Autodesk Inventor part; units mm, degrees
ref_plane "YZ Plane" through (0, 0, 0) normal (1, 0, 0) x (0, 1, 0)
ref_plane "XZ Plane" through (0, 0, 0) normal (0, 1, 0) x (-1, 0, 0)
ref_plane "XY Plane" through (0, 0, 0) normal (0, 0, 1) x (1, 0, 0)
sketch "Sketch1" plane through (0, 0, 0) normal (0, 0, 1) x (1, 0, 0)
  line L0 (-12.7, 4.7625) -> (38.1, 4.7625)
  line L1 (-15.875, -9.525) -> (44.45, -9.525)
  line L2 (-19.05, -1.5875) -> (-19.05, -26.8352)
  line L3 (44.45, -1.5875) -> (44.45, -30.4886)
  line L4 (-19.05, -9.525) -> (-15.875, -9.525)
  arc A0 (-12.7, 4.7625) -> (-19.05, -1.5875) centre (-12.7, -1.5875) ccw
  arc A1 (44.45, -1.5875) -> (38.1, 4.7625) centre (38.1, -1.5875) ccw
  line L5 (-19.05, -26.8352) -> (-19.05, -57.15)
  line L6 (-6.0043, -64.9352) -> (31.4043, -64.9352)
  line L7 (44.45, -57.15) -> (44.45, -30.4886)
  line L8 (-19.05, -57.15) -> (-14.9845, -61.2155)
  line L9 (-19.05, -57.15) -> (-13.3006, -57.15) construction
  line L10 (44.45, -57.15) -> (40.3845, -61.2155)
  line L11 (44.45, -57.15) -> (50.1994, -57.15) construction
  arc A2 (-14.9845, -61.2155) -> (-6.0043, -64.9352) centre (-6.0043, -52.2352) ccw
  arc A3 (31.4043, -64.9352) -> (40.3845, -61.2155) centre (31.4043, -52.2352) ccw
  circle A4 centre (-12.7, 0) radius 2.0955
  circle A5 centre (38.1, 0) radius 2.0955
  point P0 (0, 0)
  point P1 (25.4, 4.7625)
  point P2 (28.575, -33.6636)
  point P3 (-19.05, 4.7625)
  point P4 (44.45, 4.7625)
  point P5 (44.45, -30.1625)
  dimension "d10" = 6.35
  dimension "d13" = 45
  dimension "d14" = 135
  dimension "d15" = 12.7
  dimension "d16" = 4.191
  dimension "d17" = 4.191
extrude "Extrusion1" add sketch "Sketch1" along normal blind 1.5875
bend part "Bend Part1" radius 25.4 angle 60 line through (-15.875, -9.525, 0) along (1, 0, 0) centre toward (0, 0, 1) moving side (0, -1, 0) both sides no
equation "\"BendRadius\" = Thickness"
equation "\"BendReliefWidth\" = Thickness"
equation "\"BendReliefDepth\" = 0.5 * Thickness"
equation "\"CornerReliefSize\" = 4 * Thickness"
equation "\"MinimumRemnant\" = 2 * Thickness"
equation "\"TransitionRadius\" = BendRadius"
equation "\"JacobiRadiusSize\" = BendRadius"
equation "\"GapSize\" = Thickness"
properties part number "wedge" material "Acetal Resin, White"
Geometry: final body of the model. Coordinates: model frame, mm. A direction names the side the tool comes from. Round coordinates to 2 decimals unless told otherwise and drop trailing zeros. Loops run counter-clockwise (first coordinate to the right, second up) from the corner with the lowest first, then second, coordinate; pieces in that order, holes last. Notation, with made-up numbers: M -35,52 L 10,52 A32 ccw 10,91 Z; hole C 15.5,48 d6. An arc over 180 degrees is marked long. Put each result on its own line as item: value. Start each with the question number.
(1) Draft query along Y for faces 1 (the face through (12.256, -37.249, 25.795)), 2 (the face through (12, -2, 0)), 3 (the face through (-10.764, 0.803, 0.783)). Return one class per face: +Y half, -Y half, draft (parallel to the pull), parting line (faces both ways), or undercut.
(2) Section query D-D (x = -8.5). Return loops of the section in (y, z) (1 decimal).
(3) Section query A-A (x = 22). Return loops of the section in (y, z) (1 decimal).
(4) Material intervals for line 1 along Z through (x, y) = (36.5, -5); line 2 along Z through (x, y) = (23, -22); line 3 along Y through (x, z) = (-11, 25), sorted ascending. Write a range as [from, to].
(5) Section query B-B (y = -5). Return loops of the section in (x, z), then the cut area to 3 significant figures.
(6) Section query C-C (z = 9). Return loops of the section in (x, y), then the cut area to 3 significant figures.
(7) Set-up query: faces 4 (the face through (12, -2, 1.588)), 5 (the face through (12, 4.762, 1)). Return all of +Z, -Z, +X, -X, +Y, -Y with unobstructed straight access to the full face (end or side cutting, diameter ignored); none if empty.
(8) Contact query for flat-ended pins moving along their axis: pin 1 Ø10 at (x, z) = (13, 13) entering from +Y; pin 2 Ø6.5 at (x, y) = (-12.7, 0) entering from +Z; pin 3 Ø4 at (x, z) = (26.5, 17) entering from -Y. Output: stop coordinate, or through.
Findings below:
1. face 1: +Y half
1. face 2: draft
1. face 3: undercut
2. outline: M -45.8,37.4 L -31.5,12.7 A25.4 ccw -9.5,0 L 4.8,0 L 4.8,1.6 L -9.5,1.6 A23.8 cw -30.1,13.5 L -44.4,38.2 Z
3. outline: M -45.9,37.7 L -31.5,12.7 A25.4 ccw -9.5,0 L 4.8,0 L 4.8,1.6 L -9.5,1.6 A23.8 cw -30.1,13.5 L -44.6,38.4 Z
4. line 1: z = [0, 1.59]
4. line 2: z = [3.27, 5.12]
4. line 3: y = [-38.62, -36.79]
5. outline: M -19.05,0 L 44.45,0 L 44.45,1.59 L -19.05,1.59 Z
5. area: 101 mm2
6. outline: M -19.05,-28.92 L 44.45,-28.92 L 44.45,-26.79 L -19.05,-26.79 Z
6. area: 135 mm2
7. face 4: +Z, +X, -X, +Y
7. face 5: +Z, -Z, +X, -X, +Y
8. pin 1: stops at y = -25.78
8. pin 2: stops at z = 1.59
8. pin 3: stops at y = -35.16
